Here's how the part is built. I have some questions about the finished solid (model axes, mm). Face numbers are marked on the shaded views. A direction names the side the tool comes from. Round coordinates to 2 decimals unless told otherwise and drop trailing zeros. Write each loop counter-clockwise with the first axis right and the second up, starting at its lowest first coordinate (ties: lowest second). Pieces come first, ordered by that corner, then holes. Notation, with made-up numbers: (-38.5, 27) - (-20.5, 27) arc R15 ccw to (-20.5, 33) - close; hole circle Ø11 at (40.25, 24.5). An arc over 180 degrees is marked (long way). Use one line per item in the form item = value. Start each with the question number.
1. Will these pins go through, and if not, where does the flat tip stop? pin 1 (17 mm diameter, centred on x = -19.5, y = -5, fed in from +Z); pin 2 (8 mm diameter, centred on x = 34.5, y = -31.5, fed in from +Z); pin 3 (2 mm diameter, centred on x = -17, z = 24, fed in from +Y).
2. If I drill on line 1 along X through (y, z) = (-17.5, -14.5); line 2 along Z through (x, y) = (-20.5, 1.5); line 3 along Z through (x, y) = (-2, -3.5), over which ranges is the centre line in solid material (lowest first)?
3. I want a section at B-B, the plane y = -18. List the corners of the cut face in (x, z) for me, plus the area to 3 significant figures.
4. Which directions (+Z, -Z, +X, -X, +Y, -Y) give clear straight access to the entire face, cutting with the end or side of a thin tool? Please do the marked faces 1, 2 and 3.
5. We'd pull the mould along Z, two halves only. Please class the marked faces 4, 5 and 6: +Z half, -Z half, draft (parallel to the pull), parting line (faces both ways), or undercut.
6. I want a section at C-C, the plane x = -22. List the corners of the cut face in (y, z) for me.
7. I want a section at D-D, the plane y = -42. List the corners of the cut face in (x, z) for me.
8. I want a section at A-A, the plane z = -36. List the corners of the cut face in (x, y) for me, plus the area to 3 significant figures.
```python
from build123d import *

# Parameters (mm, degrees)
ESBO_O3_W                  = 95
ESBO_O3_H                  = 95
RESSALTO_EXTRUS_O2_DEPTH   = 47.5
CORTE_EXTRUS_O1_DEPTH      = 117.350762782
CORTE_EXTRUS_O1_DEPTH_BACK = 117.350762782
ESBO_O4_R                  = 47.5
CORTE_EXTRUS_O2_DEPTH      = 83.27241336
CORTE_EXTRUS_O2_DEPTH_BACK = 83.27241336
CORTE_EXTRUS_O3_DEPTH      = 83.27241336
CORTE_EXTRUS_O3_DEPTH_BACK = 83.27241336
ESBO_O6_W                  = 47.5
ESBO_O6_H                  = 35
ESBO_O7_W                  = 89
ESBO_O7_H                  = 41.5
CORTE_EXTRUS_O4_DEPTH      = 57


with BuildPart() as part:
    # Esboço3 → Ressalto-extrusão2 (new, symmetric)
    with BuildSketch(Plane(origin=(0, 0, 0), x_dir=(0, 0, -1), z_dir=(1, 0, 0))):
        Rectangle(ESBO_O3_W, ESBO_O3_H)
    extrude(amount=RESSALTO_EXTRUS_O2_DEPTH, both=True)

    # Esboço4 → Corte-extrusão1 (cut, two sides: drawn at the far end of the back side and taken through both)
    with BuildSketch(Plane(origin=(47.5, 0, 0), x_dir=(0, 0, -1), z_dir=(1, 0, 0)).offset(-CORTE_EXTRUS_O1_DEPTH_BACK)):
        with Locations((-47.5, 0)):
            Circle(ESBO_O4_R)
    extrude(amount=CORTE_EXTRUS_O1_DEPTH + CORTE_EXTRUS_O1_DEPTH_BACK, mode=Mode.SUBTRACT)

    # Esboço5 → Corte-extrusão2 (cut, two sides: drawn at the far end of the back side and taken through both)
    with BuildSketch(Plane(origin=(0, 0, 0), x_dir=(0, 0, -1), z_dir=(1, 0, 0)).offset(-CORTE_EXTRUS_O2_DEPTH_BACK)):
        Polygon((0, 0), (0, 47.5), (-47.5, 47.5), align=None)
    extrude(amount=CORTE_EXTRUS_O2_DEPTH + CORTE_EXTRUS_O2_DEPTH_BACK, mode=Mode.SUBTRACT)

    # Esboço6 → Corte-extrusão3 (cut, two sides: drawn at the far end of the back side and taken through both)
    with BuildSketch(Plane(origin=(0, 0, 0), x_dir=(0, 0, -1), z_dir=(1, 0, 0)).offset(-CORTE_EXTRUS_O3_DEPTH_BACK)):
        with Locations((23.75, 30)):
            Rectangle(ESBO_O6_W, ESBO_O6_H)
    extrude(amount=CORTE_EXTRUS_O3_DEPTH + CORTE_EXTRUS_O3_DEPTH_BACK, mode=Mode.SUBTRACT)

    # Esboço7 → Corte-extrusão4 (cut)
    with BuildSketch(Plane(origin=(0, 12.5, 0), x_dir=(1, 0, 0), z_dir=(0, 1, 0))):
        with Locations((0, 23.75)):
            Rectangle(ESBO_O7_W, ESBO_O7_H)
    extrude(amount=-CORTE_EXTRUS_O4_DEPTH, mode=Mode.SUBTRACT)


solid = part.part
```
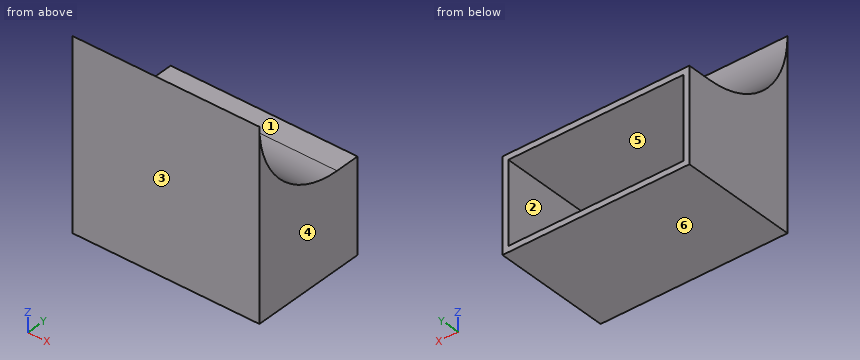
Model answer:
q1.pin_1 = 1.96
q1.pin_2 = 15.94
q1.pin_3 = -40.69
q2.line_1 = -47.5 to -44.5, 44.5 to 47.5
q2.line_2 = -47.5 to -44.5, -3 to 0
q2.line_3 = -47.5 to -44.5, -3 to 0.13
q3.outline = (-47.5, -47.5) - (47.5, -47.5) - (47.5, 3.54) - (-47.5, 3.54) - close; hole (-44.5, -44.5) - (44.5, -44.5) - (44.5, -3) - (-44.5, -3) - close
q3.area = 1,160 mm2
q4.face_1 = +Z, +X, -X, +Y
q4.face_2 = +Y
q4.face_3 = +Z, -Z, +X, -X, -Y
q5.face_4 = draft
q5.face_5 = undercut
q5.face_6 = -Z half
q6.outline = (-47.5, -47.5) - (12.5, -47.5) - (12.5, -44.5) - (-44.5, -44.5) - (-44.5, -3) - (12.5, -3) - (12.5, 0) - (0, 0) arc R47.5 cw to (-47.5, 47.5) - close
q7.outline = (-47.5, -47.5) - (47.5, -47.5) - (47.5, 25.31) - (-47.5, 25.31) - close; hole (-44.5, -44.5) - (44.5, -44.5) - (44.5, -3) - (-44.5, -3) - close
q8.outline = (-47.5, -47.5) - (47.5, -47.5) - (47.5, 12.5) - (44.5, 12.5) - (44.5, -44.5) - (-44.5, -44.5) - (-44.5, 12.5) - (-47.5, 12.5) - close
q8.area = 627 mm2
